Input: part model. Units: mm. Frame: model coordinates. Give positions to 0.01 mm unless a question says otherwise; leave off trailing zeros. Write each loop counter-clockwise with the first axis right and the second up, starting at its lowest first coordinate (ties: lowest second). Pieces come first, ordered by that corner, then holes. Notation, with made-up numbers: (88, -32) -> (139, -32) arc R28 cw to (139, -1) -> close; hole circle Ø1 at (-38.75, 30). An arc over 180 degrees is marked (long way). Return JSON: item names as keys, results as strings. Group by question number.
Item 1: Section A-A, the plane z = -299. Return loops of the section in (x, y), then the cut area to 3 significant figures.
Item 2: Line query: line 1 (Y direction, x = -51, z = -157); line 2 (Z direction, x = -67, y = 21); line 3 (Y direction, x = -75, z = -67). Output: solid intervals per line, ascending. Write a range as [from, to].
Item 3: Pin query (flat end, axial travel): P1, Ø2, axis at x = -255, z = -330, coming from the +Y side (3 decimals); P2, Ø12, axis at x = -493.5, z = -256.5, coming from the -Y side. Return the tip coordinate at first contact, or that it passes through.
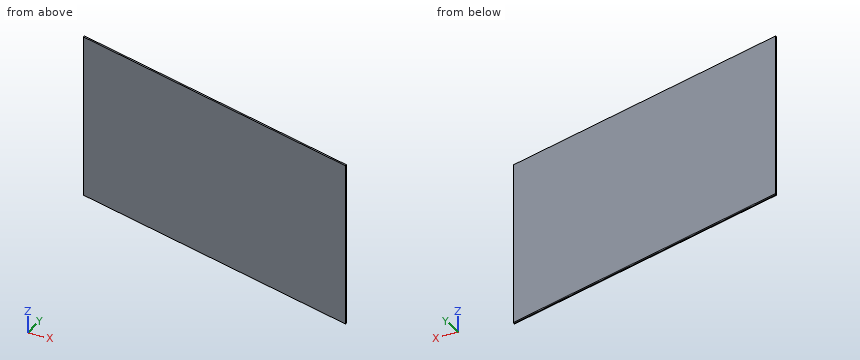
Autodesk Inventor part; units mm, degrees
ref_plane "YZ Plane" through (0, 0, 0) normal (1, 0, 0) x (0, 1, 0)
ref_plane "XZ Plane" through (0, 0, 0) normal (0, 1, 0) x (-1, 0, 0)
ref_plane "XY Plane" through (0, 0, 0) normal (0, 0, 1) x (1, 0, 0)
sketch "스케치1" plane through (0, 0, 0) normal (0, 0, 1) x (1, 0, 0)
  line L0 (0, 0) -> (0, 5)
  line L1 (0, 0) -> (-850, 227.7568)
  line L2 (-12.9463, 0) -> (8.7754, 0)
  line L3 (0, 5) -> (-850, 232.7568)
  line L4 (-850, 227.7568) -> (-850, 232.7568)
  point P0 (-850, 230.2568)
  point P1 (-850, 242.7568)
  point P2 (0, 15)
  dimension "d0" = 15
  dimension "d1" = 5
  dimension "d2" = 850
extrude "돌출1" add sketch "스케치1" against normal blind 450
sketch "스케치3" plane through (0, 15, 0) normal (0.2588, 0.9659, 0) x (0.9659, -0.2588, 0)
  line L0 (-879.9848, 0) -> (-879.9848, 450)
  line L1 (3.8823, 0) -> (3.8823, 450)
  spline S0 degree 4 poles (-879.9848, 225) (-790.3669, 315.2357) (-705.7025, 105.8229) (-615.8925, 383.2001) (-422.1913, 176.8706) (-352.8385, 360.4529) (-185.1098, 145.8092) (-106.461, 355.2219) (-47.5696, 282.9867) (3.8823, 225) knots 0 0 0 0 0 0.288179 0.401252 0.519809 0.635267 0.741109 1 1 1 1 1
  line L2 (-879.9848, 225) -> (-986.5845, 327.8412)
  line L3 (-986.5845, 327.8412) -> (-911.355, 729.5985)
  line L4 (-911.355, 729.5985) -> (113.0461, 683.1803)
  line L5 (113.0461, 683.1803) -> (3.8823, 225)
  point P0 (-751.2924, 234.868)
  point P1 (-666.4591, 234.868)
  point P2 (-560.8178, 275.0205)
  point P3 (-432.7676, 244.6086)
  point P4 (-339.9313, 291.6979)
  point P5 (-223.0855, 244.6086)
  point P6 (-138.2523, 275.0205)
  point P7 (-77.4285, 291.6979)
extrude "돌출3" [suppressed]
fillet "모깎기4" [suppressed]
fillet "모깎기5" radius 2 1 edges at (-425, 118.8784, -450)
properties part number "부품2" material "에폭시 수지"
Answer below:
{
 "1": {"outline": "(-850, 227.76) -> (0, 0) -> (0, 5) -> (-850, 232.76) -> close", "area": "4,250 mm2"},
 "2": {"line 1": "y = [13.67, 18.67]", "line 2": "z = [-450, 0]", "line 3": "y = [20.1, 25.1]"},
 "3": {"P1": "stops at y = 73.595", "P2": "stops at y = 130.63"}
}
